Geometry check sheet. Reference: the model listing, model coordinates, mm. Face numbers are marked on the shaded views. A direction names the side the tool comes from. Coordinates: 2 decimals unless noted, no trailing zeros. Write each loop counter-clockwise with the first axis right and the second up, starting at its lowest first coordinate (ties: lowest second). Pieces come first, ordered by that corner, then holes. Notation, with made-up numbers: M -12,-20 L 23,-20 A13 cw 23,0 Z; hole C 45,63 d4. An arc over 180 degrees is marked long. Put each result on its own line as item: value. Start each with the question number.
1) Gauge pin test, flat ends, axial feed: pin 1 (2.5 mm diameter, centred on x = -3, y = 4, fed in from +Z); pin 2 (1 mm diameter, centred on y = 2, z = 48.5, fed in from -X); pin 3 (12 mm diameter, centred on x = 33, z = -18, fed in from +Y); pin 4 (3 mm diameter, centred on y = 2, z = 17, fed in from -X). Record the tip position at first contact, or that the pin passes through.
2) Cross-section at C-C on x = 31. Record the cut outline in (y, z).
3) Mould release check, pull along Z, two halves, no side actions. Record for the marked faces 3, 4, 5 and 6: released by +Z, released by -Z, zero draft, split by the parting line, or undercut.
4) Scan lines: line 1 along X through (y, z) = (5.5, -9.5); line 2 along X through (y, z) = (7.75, -3); line 3 along X through (y, z) = (3.25, 7). Record each from-to range of solid material in increasing order.
5) Cross-section at A-A on y = 1.5. Record the cut outline in (x, z), plus the area to 3 significant figures.
6) Set-up check for the marked faces 1 and 2: record each of +Z, -Z, +X, -X, +Y, -Y from which the full face is reachable in a straight line by a thin tool's end or side.
7) Cross-section at B-B on z = 52. Record the cut outline in (x, y) (3 decimals).
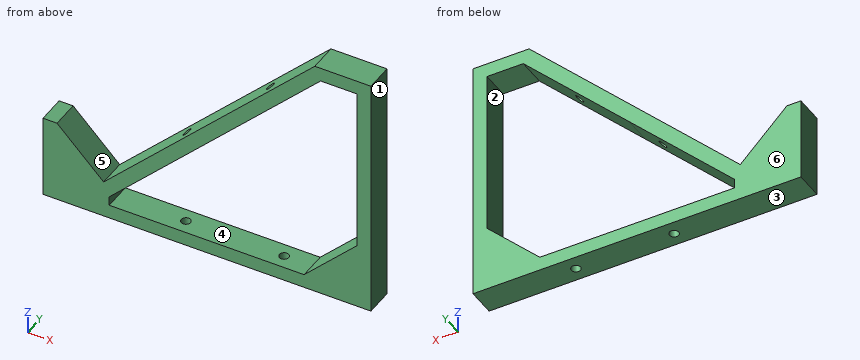
Solid Edge part; units mm, degrees
sketch "Sketch1" plane through (0, 0, 0) normal (0, -1, 0) x (1, 0, 0)
  line L0 (-5, -30) -> (-5, 0)
  line L1 (0, 0) -> (-5, 0)
  line L2 (0, 0) -> (16.617, -16.617)
  line L3 (16.617, -16.617) -> (91.9239, 58.6899)
  line L4 (91.9239, 58.6899) -> (111.9239, 58.6899)
  line L5 (111.9239, -30) -> (111.9239, 58.6899)
  line L6 (-5, -30) -> (111.9239, -30)
  line L7 (56.306, 16.0009) -> (93.9949, 53.6899)
  line L8 (93.9949, 53.6899) -> (106.9239, 53.6899)
  line L9 (106.9239, 24.3449) -> (106.9239, 53.6899)
  line L10 (106.9239, -6.1716) -> (106.9239, 24.3449)
  line L11 (97.5097, -15.5858) -> (106.9239, -6.1716)
  line L12 (97.5097, -15.5858) -> (88.0955, -25)
  line L13 (88.0955, -25) -> (52.7704, -25)
  line L14 (18.617, -25) -> (52.7704, -25)
  line L15 (18.617, -21.6881) -> (18.617, -25)
  line L16 (56.306, 16.0009) -> (18.617, -21.6881)
extrude "Protrusion1" add sketch "Sketch1" against normal blind 10
sketch "Sketch2" plane through (54.2704, 3.5, 21.0364) normal (-0.7071, 0, 0.7071) x (0.7071, 0, 0.7071)
  circle A0 centre (-15.25, 1.5) radius 1.6
  circle A1 centre (26.75, 1.5) radius 1.6
extrude "Cutout1" cut sketch "Sketch2" against normal up to next
sketch "Sketch3" plane through (53.3562, 5, -25) normal (0, 0, 1) x (1, 0, 0)
  circle A0 centre (-10.2608, 0) radius 1.65
  circle A1 centre (24.7392, 0) radius 1.65
extrude "Cutout2" cut sketch "Sketch3" against normal up to next
Answer key:
1. pin 1: stops at z = 0
1. pin 2: stops at x = 81.23
1. pin 3: passes through
1. pin 4: stops at x = 48.73
2. outline: M 0,-30 L 10,-30 L 10,-25 L 0,-25 Z; M 0,-9.31 L 10,-9.31 L 10,-2.23 L 0,-2.23 Z
3. face 3: released by -Z
3. face 4: undercut
3. face 5: released by +Z
3. face 6: zero draft
4. line 1: x = -5 to 9.5, 23.73 to 30.81, 103.6 to 111.92
4. line 2: x = -5 to 3, 30.23 to 37.31, 106.92 to 111.92
4. line 3: x = 40.23 to 47.31, 106.92 to 111.92
5. outline: M -5,-30 L 111.92,-30 L 111.92,58.69 L 91.92,58.69 L 16.62,-16.62 L 0,0 L -5,0 Z; hole M 18.62,-25 L 88.1,-25 L 106.92,-6.17 L 106.92,53.69 L 93.99,53.69 L 56.31,16 L 18.62,-21.69 Z
5. area: 2,200 mm²
6. face 1: +Z, -Z, +X, +Y, -Y
6. face 2: +Y, -Y
7. outline: M 85.234,0 L 92.305,0 L 92.305,10 L 85.234,10 Z; M 106.924,0 L 111.924,0 L 111.924,10 L 106.924,10 Z
